```python
from build123d import *

# Parameters (mm, degrees)
SKETCH1_W           = 20
SKETCH1_H           = 14
BOSS_EXTRUDE1_DEPTH = 30
SKETCH2_W           = 40
SKETCH2_H           = 40
BOSS_EXTRUDE2_DEPTH = 20
FILLET1_R           = 10


with BuildPart() as part:
    # Sketch1 → Boss-Extrude1 (new body)
    with BuildSketch(Plane.XY):
        with Locations((-20, -7)):
            Rectangle(SKETCH1_W, SKETCH1_H)
    extrude(amount=BOSS_EXTRUDE1_DEPTH)

    # Sketch2 → Boss-Extrude2 (add)
    with BuildSketch(Plane.XY):
        with Locations((-10, 6)):
            Rectangle(SKETCH2_W, SKETCH2_H)
    extrude(amount=-BOSS_EXTRUDE2_DEPTH)

    # Fillet1
    fillet1_edges = [part.edges().sort_by_distance(p)[0] for p in [
        (10, 26, -10),
        (-20, 0, 30),
        (-20, 0, 0),
    ]]
    fillet(fillet1_edges, radius=FILLET1_R)


solid = part.part
```
Work out the finished part from the listing and answer in its coordinate system (mm). A direction names the side the tool comes from. Round coordinates to 2 decimals unless told otherwise and drop trailing zeros. Write each loop counter-clockwise with the first axis right and the second up, starting at its lowest first coordinate (ties: lowest second). Pieces come first, ordered by that corner, then holes.
1) A cutting plane is placed at C-C on z = 12. Determine the outline of the cut face in (x, y), and give its area (3 significant figures).
2) Flat-ended cylindrical pins translate along their axes: P1, Ø8, axis at x = -16.5, y = 8, coming from the +Z side; P2, Ø10, axis at x = 1.5, z = -14, coming from the +Y side; P3, Ø3, axis at x = -16, z = 16.5, coming from the +Y side; P4, Ø2, axis at x = 1, y = 2.5, coming from the +Z side. Find the tip coordinate at first contact, or state that the pin passes through.
3) Consider probe 1 along Z at (x, y) = (1, 9.5); probe 2 along X at (y, z) = (-2.5, 8); probe 3 along Y at (x, z) = (-10.5, 1). Determine where each line is inside the solid, lowest interval first.
4) A cutting plane is placed at A-A on x = -21. Determine the outline of the cut face in (y, z).
5) A cutting plane is placed at B-B on y = 2. Determine the outline of the cut face in (x, z), and give its area (3 significant figures).
6) A cutting plane is placed at D-D on x = 6. Determine the outline of the cut face in (y, z), and give its area (3 significant figures).
7) Which of the six approach directions +Z, -Z, +X, -X, +Y, -Y give full straight-line access (tool end or side, diameter ignored) to faces 1 (the face through (-10, -8, 15)), 2 (the face through (-20, 0, 15)), 3 (the face through (-6, 11, 0))?
Entries:
1. outline: (-30, -14) - (-10, -14) - (-10, 0) - (-30, 0) - close
1. area: 280 mm2
2. P1: stops at z = 2
2. P2: stops at y = 26
2. P3: stops at y = 0
2. P4: stops at z = 0
3. probe 1: z = -20 to 0
3. probe 2: x = -30 to -10
3. probe 3: y = -14 to 5.64
4. outline: (-14, -20) - (26, -20) - (26, 0) - (10, 0) arc R10 cw to (0, 10) - (0, 20) arc R10 ccw to (-10, 30) - (-14, 30) - close
5. outline: (-30, -20) - (10, -20) - (10, 0) - (-10, 0) - (-10, 4) - (-30, 4) - close
5. area: 880 mm2
6. outline: (-14, -20) - (24, -20) - (24, 0) - (-14, 0) - close
6. area: 760 mm2
7. face 1: +Z, +X, +Y, -Y
7. face 2: +Z, +X, -X, +Y
7. face 3: +Z, +X, +Y
